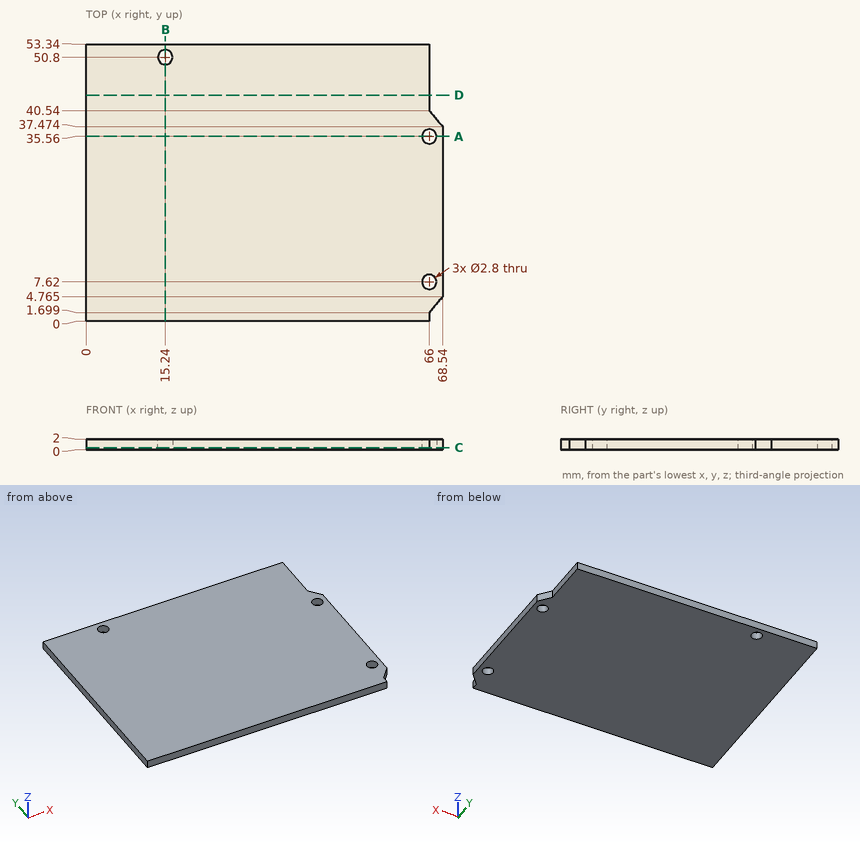
Geometry: see drawing. Coordinates: mm, zero at the bounding-box minimum. Give positions to 0.01 mm unless a question says otherwise; leave off trailing zeros. Order: outer loops, then holes, each group sorted by start corner. A loop starts at its lowest first (then second) coordinate and runs counter-clockwise, first axis right, second up. Notation, with made-up numbers: (-24.75, 54) - (13.25, 54) arc R21 ccw to (13.25, 80) - close; hole circle Ø8 at (-15, 6.5). An arc over 180 degrees is marked (long way). Use CSV: the item, a comma, the result in double quotes.
1. Section query D-D (y = 43.5). Output: boundary loops of the cut face in (x, z), plus the area to 3 significant figures.
Answers below:
outline,"(0, 0) - (66, 0) - (66, 2) - (0, 2) - close"
area,"132 mm2"
2. Contact query for a flat-ended pin moving along its axis: pin 1 (0.6 mm diameter, centred on y = 46, z = 1, fed in from +X). Output: stop coordinate, or through.
Answers below:
pin 1,"x = 66"
3. Section query A-A (y = 35.56). Output: boundary loops of the cut face in (x, z).
Answers below:
outline,"(0, 0) - (64.6, 0) - (64.6, 2) - (0, 2) - close; (67.4, 0) - (68.54, 0) - (68.54, 2) - (67.4, 2) - close"
4. Material intervals for line 1 along Y through (x, z) = (15.24, 1.5), sorted ascending. Write a range as from..to.
Answers below:
line 1,"0..49.4, 52.2..53.34"
5. Section query C-C (z = 0.45). Output: boundary loops of the cut face in (x, y) (1 decimal).
Answers below:
outline,"(0, 0) - (66, 0) - (66, 1.7) - (68.5, 4.8) - (68.5, 37.5) - (66, 40.5) - (66, 53.3) - (0, 53.3) - close; hole circle Ø2.8 at (15.2, 50.8); hole circle Ø2.8 at (66, 7.6); hole circle Ø2.8 at (66, 35.6)"
6. Section query B-B (x = 15.24). Output: boundary loops of the cut face in (y, z), plus the area to 3 significant figures.
Answers below:
outline,"(0, 0) - (49.4, 0) - (49.4, 2) - (0, 2) - close; (52.2, 0) - (53.34, 0) - (53.34, 2) - (52.2, 2) - close"
area,"101 mm2"
